from build123d import *

# Parameters (mm, degrees)
F0_W     = 50.8
F0_H     = 50.8
F0_W_2   = 38.1
F0_H_2   = 38.1
F1_DEPTH = 311.15
F3_DEPTH = 50.8
F4_R     = 5.08


with BuildPart() as f1:
    # F0 (on Front) → F1 (new body, symmetric)
    with BuildSketch(Plane.XZ):
        Rectangle(F0_W, F0_H)
        Rectangle(F0_W_2, F0_H_2, mode=Mode.SUBTRACT)
    extrude(amount=F1_DEPTH, both=True)

    # F2 (on face) → F3 (cut)
    with BuildSketch(Plane(origin=(-25.4, 0, 0), x_dir=(0, -1, 0), z_dir=(-1, 0, 0))):
        Polygon((-306.705576, 25.4), (-311.15, 25.4), (-311.15, -25.4), align=None)
    extrude(amount=-F3_DEPTH, mode=Mode.SUBTRACT)

    # F4
    f4_edges = [f1.edges().sort_by_distance(p)[0] for p in [
        (25.4, -2.222212, 25.4),
        (-25.4, -2.222212, 25.4),
        (25.4, 0, -25.4),
        (-25.4, 0, -25.4),
        (19.05, -1.944436, 19.05),
        (-19.05, -1.944436, 19.05),
        (19.05, -0.277777, -19.05),
        (-19.05, -0.277777, -19.05),
    ]]
    fillet(f4_edges, radius=F4_R)


solid = f1.part
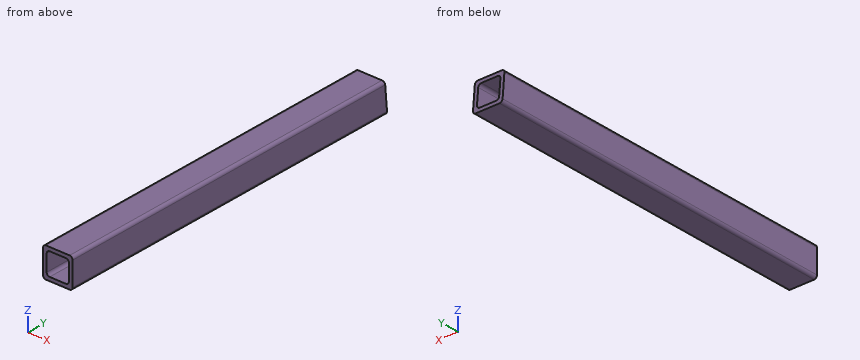
Verification items for the finished model (mm, model axes). Give positions to 0.01 mm unless a question says otherwise; leave off trailing zeros. Write each loop counter-clockwise with the first axis right and the second up, starting at its lowest first coordinate (ties: lowest second). Pieces come first, ordered by that corner, then holes. Notation, with made-up numbers: M -3,71 L 50,71 A17 ccw 50,85 Z; hole C 22.25,-9.75 d2. An arc over 180 degrees is marked long. Write item = value, one per line.
(1) Sectioned sample at A-A (x = -6). Record the cut outline in (y, z).
Found:
outline = M -311.15,-25.4 L 311.15,-25.4 L 310.59,-19.05 L -311.15,-19.05 Z; M -311.15,19.05 L 307.26,19.05 L 306.71,25.4 L -311.15,25.4 Z
(2) Sectioned sample at C-C (y = -60). Record the cut outline in (x, z), then the cut area to 3 significant figures.
Found:
outline = M -25.4,-20.32 A5.08 ccw -20.32,-25.4 L 20.32,-25.4 A5.08 ccw 25.4,-20.32 L 25.4,20.32 A5.08 ccw 20.32,25.4 L -20.32,25.4 A5.08 ccw -25.4,20.32 Z; hole M -19.05,-13.97 A5.08 ccw -13.97,-19.05 L 13.97,-19.05 A5.08 ccw 19.05,-13.97 L 19.05,13.97 A5.08 ccw 13.97,19.05 L -13.97,19.05 A5.08 ccw -19.05,13.97 Z
area = 1,130 mm2
(3) Material ranges on line 1 (Z direction, x = -7, y = -161); line 2 (Z direction, x = 14.5, y = 149), recorded low to high.
Found:
line_1 = -25.4 to -19.05, 19.05 to 25.4
line_2 = -25.4 to -19.02, 19.02 to 25.4
(4) Sectioned sample at B-B (z = -8). Record the cut outline in (x, y).
Found:
outline = M -25.4,-311.15 L -19.05,-311.15 L -19.05,309.63 L -25.4,309.63 Z; M 19.05,-311.15 L 25.4,-311.15 L 25.4,309.63 L 19.05,309.63 Z
